Read the model definition and answer for the solid it produces. Units are mm, in the model's axes. Face numbers are marked on the shaded views. Coordinates: 2 decimals unless noted, no trailing zeros. Loops run counter-clockwise (first coordinate to the right, second up) from the corner with the lowest first, then second, coordinate; pieces in that order, holes last.
Q1. Flat-ended cylindrical pins translate along their axes: P1, Ø4, axis at x = 591.5, z = -8.5, coming from the +Y side (3 decimals); P2, Ø4, axis at x = 165, z = 18.5, coming from the +Y side; P3, Ø6, axis at y = -0.5, z = 19, coming from the +X side. Find the tip coordinate at first contact, or state that the pin passes through.
Q2. The mould has two halves that part along Z. Classify the marked faces 1, 2 and 3: pulls with the +Z half, pulls with the -Z half, needs draft (parallel to the pull), parting line crosses it, or undercut.
Q3. Section B-B (x = 306) is taken. Give the vertices of the cut face in (y, z) (3 decimals).
Q4. Section A-A (z = 3) is taken. Give the vertices of the cut face in (x, y) (3 decimals), then the cut area to 3 significant figures.
Q5. Section C-C (y = 20) is taken. Give the vertices of the cut face in (x, z) (3 decimals), then the cut area to 3 significant figures.
Q6. Straight lines are drawn through the part: line 1 (Z direction, x = 276, y = -7) (3 decimals); line 2 (Y direction, x = 137, z = -3) (3 decimals); line 3 (Y direction, x = 502.5, z = 6) (3 decimals). For each, find the intervals that lie inside material, in ascending order.
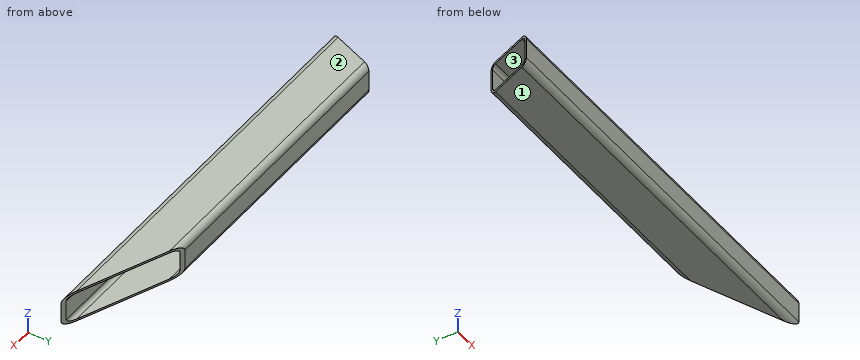
Autodesk Inventor part; units mm, degrees
ref_plane "YZ Plane" through (0, 0, 0) normal (1, 0, 0) x (0, 1, 0)
ref_plane "XZ Plane" through (0, 0, 0) normal (0, 1, 0) x (-1, 0, 0)
ref_plane "XY Plane" through (0, 0, 0) normal (0, 0, 1) x (1, 0, 0)
sketch "Sketch1" plane through (0, 0, 0) normal (1, 0, 0) x (0, 1, 0)
  line L0 (-28.575, 25.4) -> (28.575, 25.4)
  line L1 (38.1, 15.875) -> (38.1, -15.875)
  line L2 (28.575, -25.4) -> (-28.575, -25.4)
  line L3 (-38.1, -15.875) -> (-38.1, 15.875)
  line L4 (-38.1, 25.4) -> (38.1, -25.4) construction
  line L5 (38.1, 25.4) -> (-38.1, -25.4) construction
  arc A0 (38.1, 15.875) -> (28.575, 25.4) centre (28.575, 15.875) ccw
  arc A1 (-28.575, 25.4) -> (-38.1, 15.875) centre (-28.575, 15.875) ccw
  arc A2 (-38.1, -15.875) -> (-28.575, -25.4) centre (-28.575, -15.875) ccw
  arc A3 (28.575, -25.4) -> (38.1, -15.875) centre (28.575, -15.875) ccw
  line L6 (34.925, -15.875) -> (34.925, 15.875)
  arc A4 (34.925, 15.875) -> (28.575, 22.225) centre (28.575, 15.875) ccw
  line L7 (28.575, 22.225) -> (-28.575, 22.225)
  arc A5 (-28.575, 22.225) -> (-34.925, 15.875) centre (-28.575, 15.875) ccw
  line L8 (-34.925, 15.875) -> (-34.925, -15.875)
  arc A6 (-34.925, -15.875) -> (-28.575, -22.225) centre (-28.575, -15.875) ccw
  line L9 (-28.575, -22.225) -> (28.575, -22.225)
  arc A7 (28.575, -22.225) -> (34.925, -15.875) centre (28.575, -15.875) ccw
  point P0 (0, 0)
  dimension "d0" = 76.2
  dimension "d1" = 50.8
  dimension "d2" = 9.525
  dimension "d3" = 3.175
extrude "Extrusion1" add sketch "Sketch1" along normal blind 660.4
sketch "Sketch2" plane through (0, -28.575, 25.4) normal (0, 0, 1) x (1, 0, 0)
  line L0 (0, -9.525) -> (660.4, -9.525)
  line L1 (0, -9.525) -> (31.75, 66.675)
  line L2 (0, 66.675) -> (660.4, 66.675)
  line L3 (0, 57.15) -> (0, 0)
  line L4 (0, 57.15) -> (0, 66.675)
  line L5 (54.4286, 66.675) -> (0, 66.675)
  line L6 (0, 66.675) -> (0, -9.525)
  line L7 (660.4, -9.525) -> (477.52, 66.675)
  line L8 (477.52, 66.675) -> (660.4, 66.675)
  line L9 (660.4, 66.675) -> (660.4, -9.525)
  line L10 (0, 57.15) -> (660.4, 57.15)
  point P0 (0, 28.575)
  dimension "d6" = 22.62
  dimension "d7" = 22.62
extrude "Extrusion2" cut sketch "Sketch2" against normal through all contours L6 L3 L10 L1 | L7 L10 L9 | L10 L4 L2 L1 | L7 L2 L9 L10
equation "\"d0\" = stockWidth"
equation "\"d1\" = stockHeight"
equation "\"d2\" = stockRad"
equation "\"d3\" = stockGuage"
equation "\"d4\" = sup1Len"
equation "\"d6\" = sup1Ang"
equation "\"d7\" = sup1Ang"
equation "\"height\" = 203.2"
equation "\"shaftDiam\" = 6.35"
equation "\"shaftSpace\" = 1.5875"
equation "\"stageSpace\" = 2.54"
equation "\"stageAngle\" = 15deg"
equation "\"stockHeight\" = 50.8"
equation "\"stockWidth\" = 76.2"
equation "\"stockRad\" = 9.525"
equation "\"stockGuage\" = 3.175"
equation "\"groundActu\" = 304.8"
equation "\"baseWidth\" = 1066.8"
equation "\"baseDepth\" = 254"
equation "\"capThickness\" = 3.175"
equation "\"sup1Len\" = 660.4"
equation "\"sup1Ang\" = 22.6199deg"
equation "\"supVertLen\" = 955.13561"
equation "\"sup2Ang\" = 8.959949deg"
equation "\"sup2Len\" = 2079.37366"
equation "\"supSideAng\" = 19.376933deg"
equation "\"supSideLen\" = 1531.12879"
equation "\"FlangeDiam\" = 12.7"
equation "\"bearingDiam\" = 9.5504"
equation "\"FlangeDepth\" = 1.5875"
equation "\"smallFilet\" = 0.39687"
equation "\"thickness\" = 12.7"
equation "\"ringDiam\" = 96.46608"
properties part number "support 1" material "Aluminum 6061"
Numbers:
1. P1: stops at y = -34.925
1. P2: stops at y = 38.08
1. P3: passes through
2. face 1: pulls with the -Z half
2. face 2: pulls with the +Z half
2. face 3: undercut
3. outline: (-38.1, -15.875) arc R9.525 ccw to (-28.575, -25.4) - (28.575, -25.4) arc R9.525 ccw to (38.1, -15.875) - (38.1, 15.875) arc R9.525 ccw to (28.575, 25.4) - (-28.575, 25.4) arc R9.525 ccw to (-38.1, 15.875) - close; hole (-34.925, -15.875) arc R6.35 ccw to (-28.575, -22.225) - (28.575, -22.225) arc R6.35 ccw to (34.925, -15.875) - (34.925, 15.875) arc R6.35 ccw to (28.575, 22.225) - (-28.575, 22.225) arc R6.35 ccw to (-34.925, 15.875) - close
4. outline: (0, -38.1) - (660.4, -38.1) - (652.78, -34.925) - (1.323, -34.925) - close; (30.427, 34.925) - (485.14, 34.925) - (477.52, 38.1) - (31.75, 38.1) - close
4. area: 3,510 mm2
5. outline: (24.208, -25.4) - (520.96, -25.4) - (520.96, -22.225) - (24.208, -22.225) - close; (24.208, 22.225) - (520.96, 22.225) - (520.96, 25.4) - (24.208, 25.4) - close
5. area: 3,150 mm2
6. line 1: z = -25.4 to -22.225, 22.225 to 25.4
6. line 2: y = -38.1 to -34.925, 34.925 to 38.1
6. line 3: y = -38.1 to -34.925
